Print and shaded views of the part. All mm, measured from the part's lowest x, y and z. Coordinates: 2 decimals unless noted, no trailing zeros. Loops run counter-clockwise (first coordinate to the right, second up) from the corner with the lowest first, then second, coordinate; pieces in that order, holes last. Notation, with made-up numbers: M -40,36 L -8,36 A16 ccw -8,56 Z; hole C 29,42 d6. An arc over 180 degrees is marked long. Use a Markdown table: item, result. Add a question column.
1) Wall check: probe 1 along Y at (x, z) = (4.5, 0.65); probe 2 along Y at (x, z) = (19.5, 1.6); probe 3 along X at (y, z) = (5, 0.2). Give the ranges that are in metal, low to high. Write a range as from..to.
2) Band-saw the part on C-C (x = 34.5). List the corners of the cut face in (y, z).
3) Pin check, flat tip, straight feed: pin 1 Ø5 at (x, y) = (4.5, 4.5) entering from -Z. Stop position of the tip, or through.
4) Band-saw the part on A-A (y = 19.5). List the corners of the cut face in (x, z).
5) Band-saw the part on B-B (z = 1.2). List the corners of the cut face in (x, y).
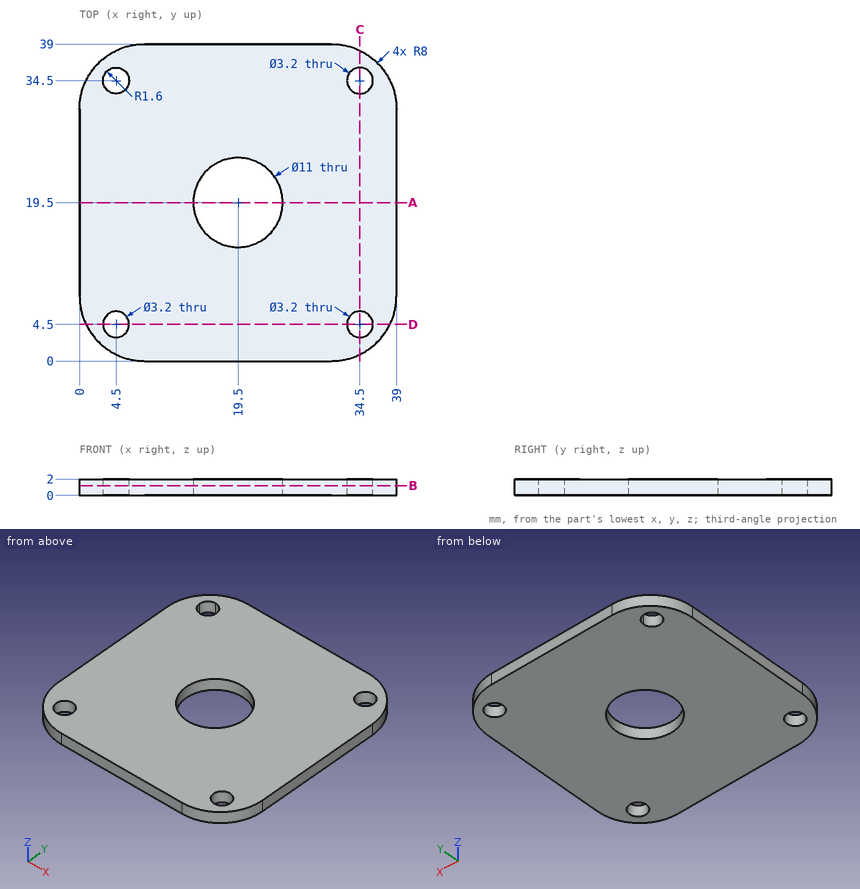
Entries:
| question | item | result |
|---|---|---|
| 1 | probe 1 | 0.81..2.9, 6.1..32.9, 36.1..38.19 |
| 1 | probe 2 | 0..14, 25..39 |
| 1 | probe 3 | 0.58..2.98, 6.02..32.98, 36.02..38.42 |
| 2 | outline | M 0.81,0 L 2.9,0 L 2.9,2 L 0.81,2 Z; M 6.1,0 L 32.9,0 L 32.9,2 L 6.1,2 Z; M 36.1,0 L 38.19,0 L 38.19,2 L 36.1,2 Z |
| 3 | pin 1 | z = 0 |
| 4 | outline | M 0,0 L 14,0 L 14,2 L 0,2 Z; M 25,0 L 39,0 L 39,2 L 25,2 Z |
| 5 | outline | M 0,8 A8 ccw 8,0 L 31,0 A8 ccw 39,8 L 39,31 A8 ccw 31,39 L 8,39 A8 ccw 0,31 Z; hole C 4.5,4.5 d3.2; hole C 4.5,34.5 d3.2; hole C 19.5,19.5 d11; hole C 34.5,4.5 d3.2; hole C 34.5,34.5 d3.2 |
